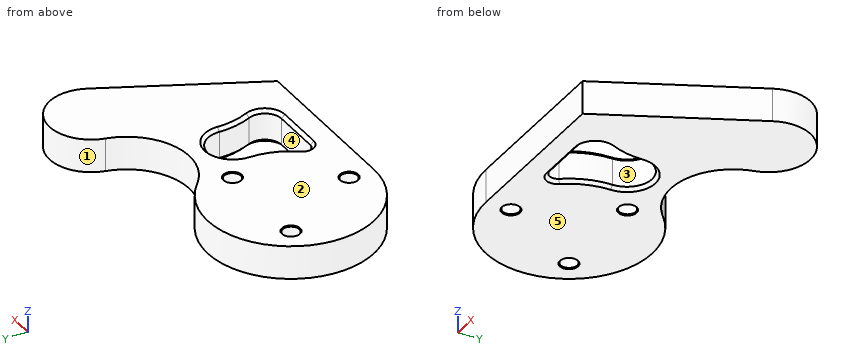
Autodesk Inventor part; units mm, degrees
ref_plane "YZ Plane" through (0, 0, 0) normal (1, 0, 0) x (0, 1, 0)
ref_plane "XZ Plane" through (0, 0, 0) normal (0, 1, 0) x (-1, 0, 0)
ref_plane "XY Plane" through (0, 0, 0) normal (0, 0, 1) x (1, 0, 0)
sketch "Sketch1" plane through (0, 0, 0) normal (0, 0, 1) x (1, 0, 0)
  arc A0 (-65.8156, 86.4888) -> (-100, 0) centre (-100, 50) ccw
  line L0 (0, 0) -> (-100, 0)
  circle A1 centre (-100, 15) radius 5
  circle A2 centre (-69.6891, 67.5) radius 5
  circle A3 centre (-130.3109, 67.5) radius 5
  arc A4 (-65.8156, 86.4888) -> (-3.6104, 105.5421) centre (-40.1774, 113.8553) ccw
  arc A5 (43.2563, 89.0796) -> (-3.6104, 105.5421) centre (20.7675, 100) ccw
  line L1 (0, 0) -> (43.2563, 89.0796)
  arc A6 (-64, 23) -> (-55, 50) centre (-100, 50) ccw
  arc A7 (-64, 23) -> (-60, 15) centre (-60, 20) ccw
  line L2 (-30, 15) -> (-60, 15)
  arc A8 (-25.0084, 49.4966) -> (-55, 50) centre (-40, 50) ccw
  arc A9 (-30, 15) -> (-20.9152, 29.1794) centre (-30, 25) ccw
  arc A10 (-25.0084, 49.4966) -> (-20.9152, 29.1794) centre (19.9662, 47.9865) ccw
  point P0 (-45, 15)
  dimension "d4" = 100
  dimension "d5" = 10
  dimension "d6" = 35
  dimension "d9" = 360
  dimension "d21" = 15
  dimension "d22" = 25
  dimension "d25" = 5
  dimension "d26" = 50
  dimension "d27" = 37.5
  dimension "d28" = 17.5
  dimension "d29" = 35
  dimension "d30" = 45
  dimension "d32" = 50
  dimension "d52" = 60
  dimension "d55" = 30
  dimension "d56" = 45
  dimension "d57" = 10
  dimension "d58" = 15
extrude "Extrusion1" add sketch "Sketch1" along normal blind 20 contours A4 A5 L1 L0 A0 | A6 A8 A10 A9 L2 A7
sketch "Sketch2" plane through (0, 0, 20) normal (0, 0, 1) x (1, 0, 0)
  arc A0 (-25.0084, 49.4966) -> (-55, 50) centre (-40, 50) ccw
  arc A1 (-25.0084, 49.4966) -> (-20.9152, 29.1794) centre (19.9662, 47.9865) ccw
  arc A2 (-64, 23) -> (-60, 15) centre (-60, 20) ccw
  arc A3 (-30, 15) -> (-20.9152, 29.1794) centre (-30, 25) ccw
  line L0 (-100, 0) -> (0, 0)
  arc A4 (-64, 23) -> (-55, 50) centre (-100, 50) ccw
  line L1 (-30, 15) -> (-60, 15)
  dimension "d65" = 50
  dimension "d69" = 30
  dimension "d70" = 15
extrude "Extrusion2" cut sketch "Sketch2" against normal blind 20
chamfer "Chamfer1" distance 2 angle 45 6 edges at (-57.3093, 35.7698, 20) (-39.7483, 64.9979, 20) (-24.1475, 39.0991, 20) (-21.58, 19.6053, 20) (-45, 15, 20) (-64.4721, 17.7639, 20)
chamfer "Chamfer2" distance 2 angle 45 6 edges at (-57.3093, 35.7698, 0) (-64.4721, 17.7639, 0) (-45, 15, 0) (-21.58, 19.6053, 0) (-24.1475, 39.0991, 0) (-39.7483, 64.9979, 0)
chamfer "Chamfer3" distance 0.5 angle 45 3 edges at (-135.3109, 67.5, 0) (-74.6891, 67.5, 0) (-105, 15, 0)
chamfer "Chamfer4" distance 0.5 angle 45 3 edges at (-74.6891, 67.5, 20) (-135.3109, 67.5, 20) (-105, 15, 20)
thread "Thread4"
thread "Thread5"
thread "Thread6"
properties part number "Curve Disc"
Geometry: final body of the model. Coordinates: model frame, mm. Face numbers are marked on the shaded views. A direction names the side the tool comes from. Give positions to 0.01 mm unless a question says otherwise; leave off trailing zeros. Loops run counter-clockwise (first coordinate to the right, second up) from the corner with the lowest first, then second, coordinate; pieces in that order, holes last. Notation, with made-up numbers: (-10.5, 82) -> (29.5, 82) arc R19 ccw to (29.5, 92) -> close; hole circle Ø7 at (-3, 49.5). An arc over 180 degrees is marked (long way). Use one line per item in the form item = value.
Item 1: Section query A-A on y = 93.5. Output: boundary loops of the cut face in (x, z), and give its area (3 significant figures).
A:
outline = (-124.65, 0) -> (-75.35, 0) -> (-75.35, 20) -> (-124.65, 20) -> close; (-8.68, 0) -> (44.91, 0) -> (44.91, 20) -> (-8.68, 20) -> close
area = 2,060 mm^2
Item 2: Section query C-C on x = -114.5. Output: boundary loops of the cut face in (y, z), and give its area (3 significant figures).
A:
outline = (2.15, 0) -> (97.85, 0) -> (97.85, 20) -> (2.15, 20) -> close
area = 1,910 mm^2
Item 3: Line query: probe 1 along Y at (x, z) = (-100, 10); probe 2 along X at (y, z) = (71, 10.5); probe 3 along Y at (x, z) = (-29.5, 5.5). Output: solid intervals per line, ascending.
A:
probe_1 = 0 to 10, 20 to 100
probe_2 = -145.38 to -133.88, -126.74 to -73.26, -66.12 to 34.48
probe_3 = 0 to 15.01, 60.71 to 77.91
Item 4: Section query B-B on z = 13.5. Output: boundary loops of the cut face in (x, y).
A:
outline = (-100, 0) -> (0, 0) -> (43.26, 89.08) arc R25 ccw (long way) to (-3.61, 105.54) arc R37.5 cw to (-65.82, 86.49) arc R50 ccw (long way) to start; hole circle Ø10 at (-130.31, 67.5); hole circle Ø10 at (-100, 15); hole circle Ø10 at (-69.69, 67.5); hole (-64, 23) arc R5 ccw to (-60, 15) -> (-30, 15) arc R10 ccw to (-20.92, 29.18) arc R45 cw to (-25.01, 49.5) arc R15 ccw (long way) to (-55, 50) arc R45 cw to start
Item 5: Access query for the marked faces 4 and 5. Directions: +Z, -Z, +X, -X, +Y, -Y. A direction counts if a zero-diameter tool reaches every point of the face in a straight line with its end or side. Return the directions, or none.
A:
face_4 = +Z, -Z
face_5 = -Z, +X, -X, +Y, -Y
Item 6: Draft query along Y for the marked faces 1, 2 and 3. Return one class per face: pulls with the +Y half, pulls with the -Y half, needs draft (parallel to the pull), parting line crosses it, or undercut.
A:
face_1 = parting line crosses it
face_2 = needs draft
face_3 = undercut
Item 7: Pin query (flat end, axial travel): P1, Ø5, axis at x = -106, z = 12, coming from the -Y side; P2, Ø4, axis at x = -79, z = 10, coming from the +Y side; P3, Ø2, axis at y = 104, z = 16, coming from the +X side; P4, Ø8, axis at x = -100, y = 15, coming from the -Z side. Return the tip coordinate at first contact, or that it passes through.
A:
P1 = 0.12
P2 = 96.25
P3 = 45.59
P4 = through
